Autodesk Inventor part; units mm, degrees
ref_plane "YZ Plane" through (0, 0, 0) normal (1, 0, 0) x (0, 1, 0)
ref_plane "XZ Plane" through (0, 0, 0) normal (0, 1, 0) x (-1, 0, 0)
ref_plane "XY Plane" through (0, 0, 0) normal (0, 0, 1) x (1, 0, 0)
sketch "Sketch1" plane through (0, 0, 0) normal (0, 0, 1) x (1, 0, 0)
  line L0 (0, 6) -> (2.75, 6)
  line L1 (2.75, 6) -> (2.75, 3)
  line L2 (2.75, 3) -> (1.5, 3)
  line L3 (1.5, 3) -> (1.5, 0)
  line L4 (1.5, 0) -> (0, 0)
  line L5 (0, 0) -> (0, 6)
  dimension "d0" = 2.75
  dimension "d1" = 3
  dimension "d2" = 3
  dimension "d3" = 1.5
revolve "Revolution1" add sketch "Sketch1" angle 360 about axis through (0, 0, 0) along (0, 1, 0)
thread "Thread1"
sketch "Sketch3" plane through (0, 6, 0) normal (0, 1, 0) x (1, 0, 0)
  line L0 (1.25, -0.7217) -> (0, -1.4434)
  line L1 (0, -1.4434) -> (-1.25, -0.7217)
  line L2 (-1.25, -0.7217) -> (-1.25, 0.7217)
  line L3 (-1.25, 0.7217) -> (0, 1.4434)
  line L4 (0, 1.4434) -> (1.25, 0.7217)
  line L5 (1.25, 0.7217) -> (1.25, -0.7217)
  point P0 (0, 0)
  point P1 (0, 0)
  dimension "d13" = 2.5
extrude "Extrusion2" cut sketch "Sketch3" against normal blind 1.5
chamfer "Chamfer2" distance 0.1 angle 45 16 edges at (0.625, 6, 1.0825) (1.25, 6, 0) (1.25, 4.5, 0) (0.625, 6, -1.0825) (0.625, 4.5, -1.0825) (-0.625, 6, -1.0825) (-0.625, 4.5, -1.0825) (-1.25, 4.5, 0) (-1.25, 6, 0) (-0.625, 4.5, 1.0825) (-0.625, 6, 1.0825) (0.625, 4.5, 1.0825) (-2.75, 6, 0) (-2.75, 3, 0) (-1.5, 3, 0) (-1.5, 0, 0)
properties part number "M3 X 3"
Geometry: final body of the model. Coordinates: model frame, mm. A direction names the side the tool comes from. Round coordinates to 2 decimals unless told otherwise and drop trailing zeros. Order: outer loops, then holes, each group sorted by start corner. A loop starts at its lowest first (then second) coordinate and runs counter-clockwise, first axis right, second up. Notation, with made-up numbers: (85.25, 7) - (101.25, 7) arc R27 ccw to (101.25, 36) - close; hole circle Ø10 at (50.25, 37.5). An arc over 180 degrees is marked (long way). Write item = value, one per line. Start each with the question number.
Q1. Cut plane C-C on y = 2.5. Return the cut outline in (x, z).
Q2. Ray query, line 1 (Y direction, x = 1.9, z = 0.4); line 2 (Z direction, x = 0.65, y = 1.25); line 3 (Y direction, x = 0.7, z = -0.15). Return the intervals inside material, ascending. Write a range as from..to.
Q3. Cut plane B-B on z = 0. Return the cut outline in (x, y), and give its area (3 significant figures).
Q4. Pull-direction query (X, two-part tool) for faces 4 (the flat face through (1.1, 6, 1.1)), 5 (the cylindrical face through (-1.5, 1.48, 0.07)), 6 (the flat face through (1.25, 5, 0)); classes: +X half, -X half, draft (parallel to the pull), parting line (faces both ways), or undercut.
Q5. Cut plane A-A on y = 5.75. Return the cut outline in (x, z), and give its area (3 significant figures).
Q6. Access query for faces 1 (the flat face through (0, 3, 2)), 2 (the flat face through (0.63, 5.26, 1.08)), 3 (the flat face through (0, 0, 0)). Directions: +Z, -Z, +X, -X, +Y, -Y. A direction counts if a zero-diameter tool reaches every point of the face in a straight line with its end or side. Return the directions, or none.
Q7. Pin query (flat end, axial travel): pin 1 (2 mm diameter, centred on x = 1.5, y = 3, fed in from -Z); pin 2 (1.2 mm diameter, centred on x = -0.5, z = 0.5, fed in from +Y). Return the tip coordinate at first contact, or that it passes through.
Outcome:
q1.outline = circle Ø3 at (0, 0)
q2.line_1 = 3..6
q2.line_2 = -1.35..1.35
q2.line_3 = 0..4.5
q3.outline = (-2.75, 3.1) - (-2.65, 3) - (-1.6, 3) - (-1.5, 2.9) - (-1.5, 0.1) - (-1.4, 0) - (1.4, 0) - (1.5, 0.1) - (1.5, 2.9) - (1.6, 3) - (2.65, 3) - (2.75, 3.1) - (2.75, 5.9) - (2.65, 6) - (1.35, 6) - (1.25, 5.9) - (1.25, 4.6) - (1.15, 4.5) - (-1.15, 4.5) - (-1.25, 4.6) - (-1.25, 5.9) - (-1.35, 6) - (-2.65, 6) - (-2.75, 5.9) - close
q3.area = 21.7 mm^2
q4.face_4 = draft
q4.face_5 = parting line
q4.face_6 = undercut
q5.outline = circle Ø5.5 at (0, 0); hole (-1.25, -0.72) - (0, -1.44) - (1.25, -0.72) - (1.25, 0.72) - (0, 1.44) - (-1.25, 0.72) - close
q5.area = 18.3 mm^2
q6.face_1 = -Y
q6.face_2 = +Y
q6.face_3 = +Z, -Z, +X, -X, -Y
q7.pin_1 = -2.7
q7.pin_2 = 5.93
